Can you work these out from the model? Positions are in its coordinate system, mm. A direction names the side the tool comes from. Coordinates: 2 decimals unless noted, no trailing zeros. Order: outer loops, then holes, each group sorted by start corner. A loop starts at its lowest first (then second) coordinate and runs counter-clockwise, first axis right, second up.
```python
from build123d import *

# Parameters (mm, degrees)
SKETCH1_R           = 14.75
SKETCH1_R_2         = 11
BOSS_EXTRUDE1_DEPTH = 7
SKETCH5_R           = 6.5
BOSS_EXTRUDE3_DEPTH = 5
FILLET2_R           = 15
CIRPATTERN2_DEPTH   = 5
CHAMFER2_SIZE       = 2
CUT_EXTRUDE3_REACH  = 54.74
CIRPATTERN4_COUNT   = 4
CUT_EXTRUDE4_REACH  = 54.967
SKETCH9_R           = 2.8
CIRPATTERN5_COUNT   = 4
CUT_EXTRUDE5_REACH  = 54.74
SKETCH10_R          = 1.6
CIRPATTERN6_COUNT   = 4


# Read off the part's stored shape, not the designer's step: CirPattern2
with BuildPart() as part:
    # Sketch1 → Boss-Extrude1 (new body)
    with BuildSketch(Plane(origin=(0, 0, 0), x_dir=(1, 0, 0), z_dir=(0, 1, 0))):
        with Locations(Location((0, 0, 0), (0, 0, 270))):
            Circle(SKETCH1_R)
        with Locations(Location((0, 0, 0), (0, 0, 270))):
            Circle(SKETCH1_R_2, mode=Mode.SUBTRACT)
    extrude(amount=BOSS_EXTRUDE1_DEPTH)

    # Sketch5 → Boss-Extrude3 (add)
    with BuildSketch(Plane.XZ):
        with BuildLine():
            ThreePointArc((6.5, 30.625), (-0.17931828, 24.127473936), (-6.49010614, 30.983500062))
            Line((-6.49010614, 30.983500062), (-7.5, 12.700885796))
            ThreePointArc((-7.5, 12.700885796), (0, 14.75), (7.5, 12.700885796))
            Line((7.5, 12.700885796), (6.49010614, 30.983500062))
            ThreePointArc((6.49010614, 30.983500062), (6.497526064, 30.80431828), (6.5, 30.625))
        make_face()
        with Locations((0, 30.625)):
            Circle(SKETCH5_R)
    extrude(amount=-BOSS_EXTRUDE3_DEPTH)

    # Fillet2
    fillet2_edges = [part.edges().sort_by_distance(p)[0] for p in [
        (7.5, 2.5, 12.700885796),
        (-7.5, 2.5, 12.700885796),
    ]]
    fillet(fillet2_edges, radius=FILLET2_R)

    # CirPattern2 outline → CirPattern2 (add)
    with BuildSketch(Plane(origin=(0, 0, 0), x_dir=(1, 0, 0), z_dir=(0, 1, 0))):
        with BuildLine():
            Line((-30.983500062, -6.49010614), (-19.060050189, -7.14873289))
            ThreePointArc((-19.060050189, -7.14873289), (-14.499104834, -8.127089257), (-10.459249152, -10.459249152))
            ThreePointArc((-10.459249152, -10.459249152), (-10.710685451, -10.156332582), (-10.969984482, -9.860118684))
            ThreePointArc((-10.969984482, -9.860118684), (0, 14.75), (10.969984482, -9.860118684))
            ThreePointArc((10.969984482, -9.860118684), (10.710685451, -10.156332582), (10.459249152, -10.459249152))
            ThreePointArc((10.459249152, -10.459249152), (14.499104834, -8.127089257), (19.060050189, -7.14873289))
            Line((19.060050189, -7.14873289), (30.983500062, -6.49010614))
            ThreePointArc((30.983500062, -6.49010614), (37.125, 0), (30.983500062, 6.49010614))
            Line((30.983500062, 6.49010614), (19.060050189, 7.14873289))
            ThreePointArc((19.060050189, 7.14873289), (14.499104834, 8.127089257), (10.459249152, 10.459249152))
            ThreePointArc((10.459249152, 10.459249152), (8.127089257, 14.499104834), (7.14873289, 19.060050189))
            Line((7.14873289, 19.060050189), (6.49010614, 30.983500062))
            ThreePointArc((6.49010614, 30.983500062), (0, 37.125), (-6.49010614, 30.983500062))
            Line((-6.49010614, 30.983500062), (-7.14873289, 19.060050189))
            ThreePointArc((-7.14873289, 19.060050189), (-8.127089257, 14.499104834), (-10.459249152, 10.459249152))
            ThreePointArc((-10.459249152, 10.459249152), (-14.499104834, 8.127089257), (-19.060050189, 7.14873289))
            Line((-19.060050189, 7.14873289), (-30.983500062, 6.49010614))
            ThreePointArc((-30.983500062, 6.49010614), (-37.125, 0), (-30.983500062, -6.49010614))
        make_face()
    extrude(amount=CIRPATTERN2_DEPTH)

    # Chamfer2
    # the kernel refuses this chamfer: 2 mm, written as the material it adds along each edge
    with BuildSketch(Plane(origin=(0, 5, 0), x_dir=(-0.7437277614936905, 0, 0.6684826226489246), z_dir=(0.6684826226489246, 0, 0.7437277614936905))) as chamfer2_piece_1_section:
        Polygon((14.75, -CHAMFER2_SIZE), (14.75 + CHAMFER2_SIZE, 0), (14.75, 0), align=None)
    chamfer2_piece_1 = revolve(axis=Axis((0, 5, 0), (0, -1, 0)), revolution_arc=263.900121289, mode=Mode.PRIVATE)
    chamfer2_piece_1 = chamfer2_piece_1 - Plane(origin=(-19.887358028, 5.976556714, 22.125900918), x_dir=(0.055153855863411774, 0, -0.998477867648251), z_dir=(0, -1, 0)) * Cylinder(15.000000014, 67, mode=Mode.PRIVATE)
    chamfer2_piece_1 = chamfer2_piece_1 - Plane(origin=(19.887358028, 5.976556714, 22.125900918), x_dir=(-0.62854059114179, 0, -0.7777767837156939), z_dir=(0, -1, 0)) * Cylinder(15.000000014, 67, mode=Mode.PRIVATE)
    chamfer2_piece_1 = chamfer2_piece_1 - Plane(origin=(22.125900918, 5.976556714, -19.887358028), x_dir=(-0.7777767837156939, 0, 0.62854059114179), z_dir=(0, -1, 0)) * Cylinder(15.000000014, 67, mode=Mode.PRIVATE)
    chamfer2_piece_1 = chamfer2_piece_1 - Plane(origin=(-19.887358028, 5.976556714, -22.125900918), x_dir=(0.62854059114179, 0, 0.7777767837156939), z_dir=(0, -1, 0)) * Cylinder(15.000000014, 67, mode=Mode.PRIVATE)
    add(chamfer2_piece_1)
    with BuildSketch(Plane(origin=(0, 5, 0), x_dir=(-0.7437277614936905, 0, 0.6684826226489246), z_dir=(0.6684826226489246, 0, 0.7437277614936905))) as chamfer2_piece_2_section:
        Polygon((14.75, -CHAMFER2_SIZE), (14.75 + CHAMFER2_SIZE, 0), (14.75, 0), align=None)
    chamfer2_piece_2 = revolve(axis=Axis((0, 5, 0), (0, -1, 0)), revolution_arc=263.900121289, mode=Mode.PRIVATE)
    chamfer2_piece_2 = chamfer2_piece_2 - Plane(origin=(-19.887358028, 5.654995073, 22.125900918), x_dir=(0.055153855863411774, 0, -0.998477867648251), z_dir=(0, -1, 0)) * Cylinder(15.000000014, 67, mode=Mode.PRIVATE)
    chamfer2_piece_2 = chamfer2_piece_2 - Plane(origin=(19.887358028, 5.654995073, 22.125900918), x_dir=(-0.62854059114179, 0, -0.7777767837156939), z_dir=(0, -1, 0)) * Cylinder(15.000000014, 67, mode=Mode.PRIVATE)
    chamfer2_piece_2 = chamfer2_piece_2 - Plane(origin=(19.887358028, 5.654995073, -22.125900918), x_dir=(-0.055153855863411774, 0, 0.998477867648251), z_dir=(0, -1, 0)) * Cylinder(15.000000014, 67, mode=Mode.PRIVATE)
    chamfer2_piece_2 = chamfer2_piece_2 - Plane(origin=(-22.125900918, 5.654995073, -19.887358028), x_dir=(0.998477867648251, 0, 0.055153855863411774), z_dir=(0, -1, 0)) * Cylinder(15.000000014, 67, mode=Mode.PRIVATE)
    add(chamfer2_piece_2)
    with BuildSketch(Plane(origin=(0, 5, 0), x_dir=(0, 0, 1), z_dir=(-1, 0, 0))) as chamfer2_piece_3_section:
        Polygon((14.75, CHAMFER2_SIZE), (14.75 + CHAMFER2_SIZE, 0), (14.75, 0), align=None)
    chamfer2_piece_3 = revolve(axis=Axis((0, 5, 0), (0, 1, 0)), revolution_arc=48.049939357, mode=Mode.PRIVATE)
    chamfer2_piece_3 = chamfer2_piece_3 - Plane(origin=(22.125900905, 5.691339401, 19.887358023), x_dir=(-0.7437277615096491, 0, -0.6684826226311694), z_dir=(0, 1, 0)) * Cylinder(15, 68, mode=Mode.PRIVATE)
    add(chamfer2_piece_3)
    with BuildSketch(Plane(origin=(0, 5, 0), x_dir=(0, 0, 1), z_dir=(-1, 0, 0))) as chamfer2_piece_4_section:
        Polygon((14.75, CHAMFER2_SIZE), (14.75 + CHAMFER2_SIZE, 0), (14.75, 0), align=None)
    chamfer2_piece_4 = revolve(axis=Axis((0, 5, 0), (0, 1, 0)), revolution_arc=48.049939357, mode=Mode.PRIVATE)
    chamfer2_piece_4 = chamfer2_piece_4 - Plane(origin=(19.887358028, 5.96883772, 22.125900918), x_dir=(-0.62854059114179, 0, -0.7777767837156939), z_dir=(0, -1, 0)) * Cylinder(15.000000014, 68, mode=Mode.PRIVATE)
    add(chamfer2_piece_4)
    with BuildSketch(Plane(origin=(0, 5, 0), x_dir=(-0.743727761509649, 0, 0.6684826226311695), z_dir=(-0.6684826226311695, 0, -0.743727761509649))) as chamfer2_piece_5_section:
        Polygon((14.75, CHAMFER2_SIZE), (14.75 + CHAMFER2_SIZE, 0), (14.75, 0), align=None)
    chamfer2_piece_5 = revolve(axis=Axis((0, 5, 0), (0, 1, 0)), revolution_arc=48.049939357, mode=Mode.PRIVATE)
    chamfer2_piece_5 = chamfer2_piece_5 - Plane(origin=(-22.125900905, 5.99378233, 19.887358023), x_dir=(0.7437277615096493, 0, -0.6684826226311694), z_dir=(0, 1, 0)) * Cylinder(15, 67, mode=Mode.PRIVATE)
    add(chamfer2_piece_5)
    with BuildSketch(Plane(origin=(0, 5, 0), x_dir=(-0.743727761509649, 0, 0.6684826226311695), z_dir=(-0.6684826226311695, 0, -0.743727761509649))) as chamfer2_piece_6_section:
        Polygon((14.75, CHAMFER2_SIZE), (14.75 + CHAMFER2_SIZE, 0), (14.75, 0), align=None)
    chamfer2_piece_6 = revolve(axis=Axis((0, 5, 0), (0, 1, 0)), revolution_arc=48.049939357, mode=Mode.PRIVATE)
    chamfer2_piece_6 = chamfer2_piece_6 - Plane(origin=(-19.887358028, 5.968837515, 22.125900918), x_dir=(0.055153855863411774, 0, -0.998477867648251), z_dir=(0, -1, 0)) * Cylinder(15.000000014, 67, mode=Mode.PRIVATE)
    add(chamfer2_piece_6)

    # Sketch8 → Cut-Extrude3 (cut, up to next)
    with BuildSketch(Plane(origin=(0, 5, 0), x_dir=(1, 0, 0), z_dir=(0, 1, 0)), mode=Mode.PRIVATE) as cut_extrude3_sk1:
        with BuildLine():
            Line((-1.55, 29.875), (-1.55, 31.375))
            ThreePointArc((-1.55, 31.375), (0, 32.925), (1.55, 31.375))
            Line((1.55, 31.375), (1.55, 29.875))
            ThreePointArc((1.55, 29.875), (0, 28.325), (-1.55, 29.875))
        make_face()
    cut_extrude3_tool1 = extrude(cut_extrude3_sk1.sketch, amount=-CUT_EXTRUDE3_REACH, mode=Mode.PRIVATE) & part.part
    cut_extrude3 = cut_extrude3_tool1.solids().sort_by_distance((0, 5, -30.625))[0]
    add(cut_extrude3, mode=Mode.SUBTRACT)

    # CirPattern4: Cut-Extrude3 ×4 about axis
    cirpattern4_axis = Axis((0, 0, 0), (0, 1, 0))
    for i in range(1, CIRPATTERN4_COUNT):
        add(cut_extrude3.rotate(cirpattern4_axis, i * 360 / CIRPATTERN4_COUNT), mode=Mode.SUBTRACT)

    # Sketch9 → Cut-Extrude4 (cut, up to next)
    with BuildSketch(Plane(origin=(0, 7, 0), x_dir=(1, 0, 0), z_dir=(0, 1, 0)), mode=Mode.PRIVATE) as cut_extrude4_sk1:
        with Locations(Location((0, 15, 0), (0, 0, 270))):
            Circle(SKETCH9_R)
    cut_extrude4_tool1 = extrude(cut_extrude4_sk1.sketch, amount=-CUT_EXTRUDE4_REACH, mode=Mode.PRIVATE) & part.part
    cut_extrude4 = cut_extrude4_tool1.solids().sort_by_distance((0, 7, -15))[0]
    add(cut_extrude4, mode=Mode.SUBTRACT)

    # CirPattern5: Cut-Extrude4 ×4 about axis
    cirpattern5_axis = Axis((0, 0, 0), (0, 1, 0))
    for i in range(1, CIRPATTERN5_COUNT):
        add(cut_extrude4.rotate(cirpattern5_axis, i * 360 / CIRPATTERN5_COUNT), mode=Mode.SUBTRACT)

    # Sketch10 → Cut-Extrude5 (cut, up to next)
    with BuildSketch(Plane(origin=(0, 5, 0), x_dir=(1, 0, 0), z_dir=(0, 1, 0)), mode=Mode.PRIVATE) as cut_extrude5_sk1:
        with Locations(Location((0, 23, 0), (0, 0, 270))):
            Circle(SKETCH10_R)
    cut_extrude5_tool1 = extrude(cut_extrude5_sk1.sketch, amount=-CUT_EXTRUDE5_REACH, mode=Mode.PRIVATE) & part.part
    cut_extrude5 = cut_extrude5_tool1.solids().sort_by_distance((0, 5, -23))[0]
    add(cut_extrude5, mode=Mode.SUBTRACT)

    # CirPattern6: Cut-Extrude5 ×4 about axis
    cirpattern6_axis = Axis((0, 0, 0), (0, 1, 0))
    for i in range(1, CIRPATTERN6_COUNT):
        add(cut_extrude5.rotate(cirpattern6_axis, i * 360 / CIRPATTERN6_COUNT), mode=Mode.SUBTRACT)


solid = part.part
```
1. I'm going to push flat-ended pins straight in: pin 1 (3 mm diameter, centred on x = 23, z = 0, fed in from +Y); pin 2 (8 mm diameter, centred on x = -24, z = -1, fed in from +Y); pin 3 (1.2 mm diameter, centred on x = 30.5, y = 2, fed in from +Z); pin 4 (2 mm diameter, centred on y = 2, z = -18, fed in from +X). Where does each tip first touch, or does it pass through?
Completed:
pin 1: passes through
pin 2: stops at y = 5
pin 3: stops at z = 6.55
pin 4: stops at x = 7.41
2. Thinking about a two-plate mould opening in Z: for faces 1 (the cylindrical face through (0.138, 2.465, 37.124)), 2 (the cylindrical face through (37.124, 2.465, 0.138)), 3 (the cylindrical face through (12.33, 3.55, 0.84)), which applies, pulls with the +Z half, pulls with the -Z half, needs draft (parallel to the pull), parting line crosses it, or undercut?
Completed:
face 1: pulls with the +Z half
face 2: parting line crosses it
face 3: undercut
3. Imagine slicing it at A-A on z = 0. Give the number of separate pieces and of enclosed holes in the cut face, then the cut area to 3 significant figures.
Completed:
separate pieces: 8
enclosed holes: 0
area: 132 mm2
4. On a 3-axis mill with a long thin cutter (end or side, diameter ignored), from which of +Z, -Z, +X, -X, +Y, -Y can I reach the whole of each face in a straight line? I mean faces 4 (the cylindrical face through (28.325, 2.535, 0.034)), 5 (the conical face through (8.793, 6.875, 11.998)). Say none if no direction works.
Completed:
face 4: +Y, -Y
face 5: +Z, +X, +Y
5. Imagine slicing it at C-C on z = 23. Please give me the cut outline in (x, y), then the cut area to 3 significant figures.
Completed:
outline: (-6.93, 0) - (-1.6, 0) - (-1.6, 5) - (-6.93, 5) - close; (1.6, 0) - (6.93, 0) - (6.93, 5) - (1.6, 5) - close
area: 53.3 mm2
6. Imagine slicing it at B-B on x = -23. Please give me the cut outline in (y, z).
Completed:
outline: (0, -6.93) - (5, -6.93) - (5, -1.6) - (0, -1.6) - close; (0, 1.6) - (5, 1.6) - (5, 6.93) - (0, 6.93) - close
7. Please list where these lines run through material, in increasing order: probe 1 along X at (y, z) = (1.45, 23); probe 2 along Z at (x, y) = (-22, 0.75); probe 3 along X at (y, z) = (2, 15).
Completed:
probe 1: x = -6.93 to -1.6, 1.6 to 6.93
probe 2: z = -6.99 to -1.25, 1.25 to 6.99
probe 3: x = -7.94 to -2.8, 2.8 to 7.94
